The drawing under review shows one solid part. Ordinate dimensions are in mm from its lowest x, y, z. A direction names the side the tool comes from. Coordinates: 2 decimals unless noted, no trailing zeros. Write each loop counter-clockwise with the first axis right and the second up, starting at its lowest first coordinate (ties: lowest second). Pieces come first, ordered by that corner, then holes. Notation, with made-up numbers: (-25.75, 41) -> (-11.75, 41) arc R9 cw to (-11.75, 54) -> close; hole circle Ø10 at (-15.75, 3). An arc over 180 degrees is marked (long way). One line per item, written item: value. Start each with the question number.
1) Add section B-B (x = 45.5). State the section outline as (y, z) points, and give its area (3 significant figures).
2) Add section D-D (z = 7). State the section outline as (x, y) points, and give its area (3 significant figures).
3) Mouldability with a two-part tool opening along X and no side actions: class the marked faces 1, 2 and 3 as released by +X, released by -X, zero draft, split by the parting line, or undercut.
4) For pin 1 Ø8 at (x, y) = (87, 5.5) entering from -Z; pin 2 Ø1 at (x, y) = (60.5, 8.5) entering from +Z; pin 3 Ø2 at (x, y) = (53.5, 37) entering from +Z, all flat-tipped, find the tip position at first contact; note any pin that passes through.
5) Add section A-A (z = 25.5). State the section outline as (x, y) points, and give its area (3 significant figures).
6) Machinability: for the marked faces 4 and 5, which of the approach directions +Z, -Z, +X, -X, +Y, -Y give a long, thin tool a straight path to every point of the face, cutting with its end or side? Answer none if there is none.
7) Add section C-C (y = 41). State the section outline as (x, z) points, and give its area (3 significant figures).
8) For probe 1 along Z at (x, y) = (46.5, 32); probe 2 along X at (y, z) = (20, 8); probe 3 along X at (y, z) = (2, 12.5), list the stretches that pass through material, from the lowest coordinate up. Write a range as from..to.
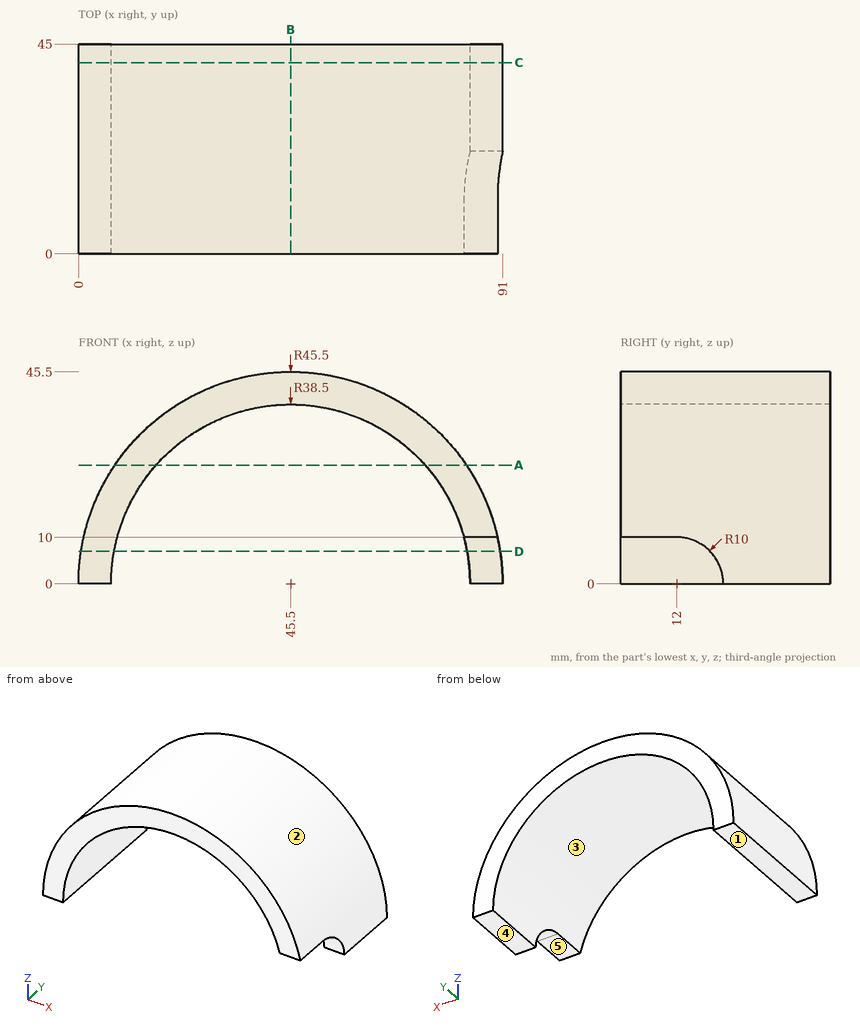
Numbers:
1. outline: (0, 38.5) -> (45, 38.5) -> (45, 45.5) -> (0, 45.5) -> close
1. area: 315 mm²
2. outline: (0.54, 0) -> (7.64, 0) -> (7.64, 45) -> (0.54, 45) -> close; (83.36, 19.14) -> (90.46, 19.14) -> (90.46, 45) -> (83.36, 45) -> close
2. area: 503 mm²
3. face 1: zero draft
3. face 2: split by the parting line
3. face 3: undercut
4. pin 1: z = 10
4. pin 2: z = 43.13
4. pin 3: z = 44.96
5. outline: (7.82, 0) -> (16.66, 0) -> (16.66, 45) -> (7.82, 45) -> close; (74.34, 0) -> (83.18, 0) -> (83.18, 45) -> (74.34, 45) -> close
5. area: 795 mm²
6. face 4: -Z, +X, -X, +Y, -Y
6. face 5: -Z, +X, -Y
7. outline: (0, 0) -> (7, 0) arc R38.5 cw to (84, 0) -> (91, 0) arc R45.5 ccw to start
7. area: 924 mm²
8. probe 1: 38.49..45.49
8. probe 2: 0.71..7.84, 83.16..90.29
8. probe 3: 1.75..9.09, 81.91..89.25
